Part model, mm, in its own coordinate system. Face numbers are marked on the shaded views. A direction names the side the tool comes from. Give positions to 0.01 mm unless a question says otherwise; leave off trailing zeros. Order: outer loops, then holes, each group sorted by start corner. A loop starts at its lowest first (then second) coordinate and runs counter-clockwise, first axis right, second up. Notation, with made-up numbers: M 6,79 L 54,79 A28 cw 54,109 Z; hole C 83,15.25 d3. An arc over 180 degrees is marked long. Return JSON: item names as keys, results as strings.
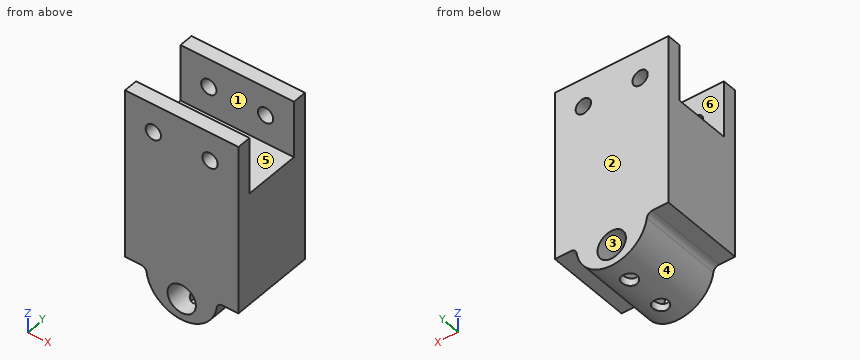
from build123d import *

# Parameters (mm, degrees)
SKETCH1_R           = 6.35
BOSS_EXTRUDE1_DEPTH = 38.1
SKETCH6_W           = 25.4
SKETCH6_H           = 25.4
CUT_EXTRUDE3_DEPTH  = 50.8
SKETCH7_R           = 3.429
CUT_EXTRUDE4_DEPTH  = 71.781852371
FILLET1_R           = 2.54
SKETCH10_R          = 3.429
CUT_EXTRUDE5_DEPTH  = 47.752


with BuildPart() as part:
    # Sketch1 → Boss-Extrude1 (new body)
    with BuildSketch(Plane(origin=(0, 0, 0), x_dir=(1, 0, 0), z_dir=(0, 1, 0))):
        with BuildLine():
            Line((-25.4, 38.1), (-15.875, 38.1))
            ThreePointArc((-15.875, 38.1), (0, 53.975), (15.875, 38.1))
            Line((15.875, 38.1), (25.4, 38.1))
            Line((25.4, 38.1), (25.4, -38.1))
            Line((25.4, -38.1), (-25.4, -38.1))
            Line((-25.4, -38.1), (-25.4, 38.1))
        make_face()
        with Locations(Location((0, 44.45, 0), (0, 0, 270))):
            Circle(SKETCH1_R, mode=Mode.SUBTRACT)
    extrude(amount=-BOSS_EXTRUDE1_DEPTH)

    # Sketch6 → Cut-Extrude3 (cut)
    with BuildSketch(Plane.ZY.offset(25.4)):
        with Locations((25.4, -19.05)):
            Rectangle(SKETCH6_W, SKETCH6_H)
    extrude(amount=-CUT_EXTRUDE3_DEPTH, mode=Mode.SUBTRACT)

    # Sketch7 → Cut-Extrude4 (cut, through all)
    with BuildSketch(Plane(origin=(0, -38.1, 0), x_dir=(-1, 0, 0), z_dir=(0, -1, 0))):
        with Locations(Location((12.7, -25.4, 0), (0, 0, 90))):
            Circle(SKETCH7_R)
        with Locations(Location((-12.7, -25.4, 0), (0, 0, 90))):
            Circle(SKETCH7_R)
    extrude(amount=-CUT_EXTRUDE4_DEPTH, mode=Mode.SUBTRACT)

    # Fillet1
    fillet1_edges = [part.edges().sort_by_distance(p)[0] for p in [
        (-15.875, -19.05, -38.1),
        (15.875, -19.05, -38.1),
    ]]
    fillet(fillet1_edges, radius=FILLET1_R)

    # Sketch10 → Cut-Extrude5 (cut)
    with BuildSketch(Plane.XY.offset(-88.9)):
        with Locations(Location((0, -27.94, 0), (0, 0, 180))):
            Circle(SKETCH10_R)
        with Locations(Location((0, -10.16, 0), (0, 0, 180))):
            Circle(SKETCH10_R)
    extrude(amount=CUT_EXTRUDE5_DEPTH, mode=Mode.SUBTRACT)


solid = part.part
Q1. Band-saw the part on B-B (x = 0). Give the cut face in (y, z) (3 decimals), then the cut area to 3 significant figures.
Established:
{"outline": "M -38.1,-53.975 L -31.369,-53.975 L -31.369,-50.8 L -38.1,-50.8 Z; M -38.1,-38.1 L 0,-38.1 L 0,38.1 L -6.35,38.1 L -6.35,12.7 L -31.75,12.7 L -31.75,38.1 L -38.1,38.1 Z; M -24.511,-53.975 L -13.589,-53.975 L -13.589,-50.8 L -24.511,-50.8 Z; M -6.731,-53.975 L 0,-53.975 L 0,-50.8 L -6.731,-50.8 Z", "area": "2,340 mm²"}
Q2. Two-plate mould, pull along Z, no slides. Class the marked faces 3, 4, 5 and 6: +Z half, -Z half, draft (parallel to the pull), parting line (faces both ways), or undercut.
Established:
{"face 3": "undercut", "face 4": "-Z half", "face 5": "+Z half", "face 6": "draft"}
Q3. Band-saw the part on A-A (z = 25.4). Give the cut face in (x, y).
Established:
{"outline": "M -25.4,-38.1 L -16.13,-38.1 L -16.13,-31.75 L -25.4,-31.75 Z; M -25.4,-6.35 L -16.13,-6.35 L -16.13,0 L -25.4,0 Z; M -9.27,-38.1 L 9.27,-38.1 L 9.27,-31.75 L -9.27,-31.75 Z; M -9.27,-6.35 L 9.27,-6.35 L 9.27,0 L -9.27,0 Z; M 16.13,-38.1 L 25.4,-38.1 L 25.4,-31.75 L 16.13,-31.75 Z; M 16.13,-6.35 L 25.4,-6.35 L 25.4,0 L 16.13,0 Z"}
Q4. Pin check, flat tips, straight feed: pin 1 (11 mm diameter, centred on x = 12.7, z = 25.4, fed in from +Y); pin 2 (5.5 mm diameter, centred on x = 0, y = -27.94, fed in from +Z); pin 3 (6 mm diameter, centred on x = 12.7, z = 25.4, fed in from +Y); pin 4 (5.5 mm diameter, centred on x = 21.5, y = -9.5, fed in from -Z). Stop position of each tip, or through.
Established:
{"pin 1": "stops at y = 0", "pin 2": "stops at z = 12.7", "pin 3": "passes through", "pin 4": "stops at z = -38.1"}
Q5. Probe line 1 along X through (y, z) = (-36.5, 25.4); line 2 along X through (y, z) = (-27.94, -51.65); line 3 along Z through (x, y) = (21, -6). List the from-to ranges inside material, lowest first.
Established:
{"line 1": "x = -25.4 to -16.13, -9.27 to 9.27, 16.13 to 25.4", "line 2": "x = -8.27 to -3.43, 3.43 to 8.27", "line 3": "z = -38.1 to 38.1"}
Q6. Band-saw the part on C-C (z = -44.45). Give the cut face in (x, y).
Established:
{"outline": "M -14.55,-38.1 L -6.35,-38.1 L -6.35,0 L -14.55,0 Z; M 6.35,-38.1 L 14.55,-38.1 L 14.55,0 L 6.35,0 Z"}
Q7. Band-saw the part on D-D (x = 12.7). Give the cut face in (y, z) (3 decimals).
Established:
{"outline": "M -38.1,-47.625 L 0,-47.625 L 0,21.971 L -6.35,21.971 L -6.35,12.7 L -31.75,12.7 L -31.75,21.971 L -38.1,21.971 Z; M -38.1,28.829 L -31.75,28.829 L -31.75,38.1 L -38.1,38.1 Z; M -6.35,28.829 L 0,28.829 L 0,38.1 L -6.35,38.1 Z"}
Q8. 3-axis set-ups, long thin cutter, end or side, ignore diameter. For the marked faces 1 and 2: which of +Z, -Z, +X, -X, +Y, -Y reach the whole face in a straight line?
Established:
{"face 1": "+Z, +X, -X", "face 2": "+Z, -Z, +X, -X, +Y"}
